Design review of the part built by this model. Coordinates are the model's own, in mm. Face numbers are marked on the shaded views. A direction names the side the tool comes from. Round coordinates to 2 decimals unless told otherwise and drop trailing zeros. Order: outer loops, then holes, each group sorted by start corner. A loop starts at its lowest first (then second) coordinate and runs counter-clockwise, first axis right, second up.
Autodesk Inventor part; units mm, degrees
ref_plane "YZ Plane" through (0, 0, 0) normal (1, 0, 0) x (0, 1, 0)
ref_plane "XZ Plane" through (0, 0, 0) normal (0, 1, 0) x (-1, 0, 0)
ref_plane "XY Plane" through (0, 0, 0) normal (0, 0, 1) x (1, 0, 0)
sketch "Sketch1" plane through (0, 0, 0) normal (0, 1, 0) x (-1, 0, 0)
  circle A0 centre (-11.43, -21.12) radius 0.25
  circle A1 centre (-11.43, -28.88) radius 0.25
  circle A2 centre (-9, -34.5) radius 1.25
  line L0 (11.43, -28.88) -> (-11.43, -28.88) construction
  circle A3 centre (11.43, -21.12) radius 0.25
  circle A4 centre (11.43, -28.88) radius 0.25
  arc A5 (-17.5, -24) -> (17.5, -24) centre (0, -24) ccw
  circle A6 centre (11.43, 2.12) radius 0.25
  circle A7 centre (-11.43, 9.88) radius 0.25
  circle A8 centre (11.43, 9.88) radius 0.25
  circle A9 centre (-9, 15.5) radius 1.25
  arc A10 (17.5, 5) -> (-17.5, 5) centre (0, 5) ccw
  circle A11 centre (-11.43, 2.12) radius 0.25
  circle A12 centre (12, -9.5) radius 1.25
  line L1 (17.5, -24) -> (17.5, 5)
  line L2 (11.43, -21.12) -> (11.43, 2.12) construction
  line L3 (0, -24) -> (0, 5) construction
  line L4 (-17.5, 5) -> (-17.5, -24)
  line L5 (-9, -34.5) -> (-9, 15.5) construction
  circle A13 centre (0, 0) radius 2.75
  point P0 (0, -41.5)
  point P1 (0, -28.88)
  point P2 (0, 22.5)
  point P3 (-9, -9.5)
  point P4 (11.43, -9.5)
  point P5 (0, -9.5)
  dimension "d0" = 17.5
  dimension "d2" = 5.5
  dimension "d3" = 64
  dimension "d4" = 2.5
  dimension "d5" = 12
  dimension "d6" = 50
  dimension "d7" = 9
  dimension "d8" = 22.86
  dimension "d9" = 7.76
  dimension "d10" = 7.76
  dimension "d11" = 23.24
  dimension "d12" = 0.5
  dimension "d13" = 9.5
extrude "Extrusion1" add sketch "Sketch1" against normal blind 9.2 contours A0 | A1 | A2 | A3 | A4 | L4 A10 L1 A5 | A6 | A7 | A8 | A9 | A11 | A12 | A13
chamfer "Chamfer1" distance 4 distance2 5 4 edges at (0, -9.2, 22.5) (-17.5, -9.2, -9.5) (0, -9.2, -41.5) (17.5, -9.2, -9.5) measured on face at (-5.8333, -9.2, -14.3333)
extrude "Extrusion2" add sketch "Sketch1" along normal blind 2.8 contours A0 | A1 | A3 | A4 | A6 | A7 | A8 | A11
extrude "Extrusion3" add sketch "Sketch1" along normal blind 3.8 contours A2 | A9 | A12
chamfer "Chamfer2" distance 0.2 angle 45 3 edges at (-10.75, 3.8, -9.5) (10.25, 3.8, 15.5) (10.25, 3.8, -34.5)
extrude "Extrusion4" add sketch "Sketch1" along normal blind 6.4 contours A13
chamfer "Chamfer3" distance 0.25 distance2 6.4 1 edges at (2.75, 6.4, 0) measured on face at (-0.9684, 6.4, -0.426)
sketch "Sketch3" plane through (0, 6.4, 0) normal (0, 1, 0) x (1, 0, 0)
  circle A0 centre (0, 0) radius 2
  dimension "d31" = 4
extrude "Extrusion5" add sketch "Sketch3" along normal blind 4.8
sketch "Sketch4" plane through (0, 11.2, 0) normal (0, 1, 0) x (1, 0, 0)
  circle A0 centre (0, 0) radius 1
  dimension "d34" = 2
extrude "Extrusion6" add sketch "Sketch4" along normal blind 6.2
chamfer "Chamfer4" distance 0.25 angle 45 1 edges at (-1, 17.4, 0)
properties part number "BKA" material "ABS Plastic"
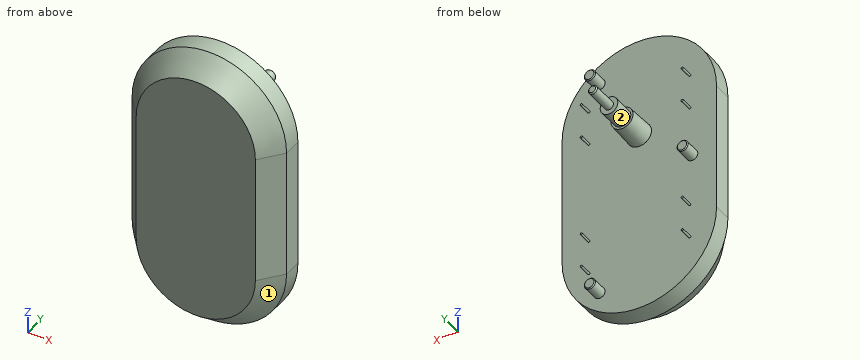
1) Take a section at B-B on y = -2. Give the boundary of the cut face in (x, z).
Results:
outline: (-17.5, -24) arc R17.5 ccw to (17.5, -24) - (17.5, 5) arc R17.5 ccw to (-17.5, 5) - close
2) For the marked faces 1 and 2, list the 3-axis set-ups (+Z, -Z, +X, -X, +Y, -Y) from which the entire face can be reached by the end or side of a thin tool; tool diameter is ignored.
Results:
face 1: -Z, -Y
face 2: +Y
3) To check wall thickness, follow line 1 along Y through (x, z) = (-2, -11); line 2 along X through (y, z) = (-7, -1.5); line 3 along Y through (x, z) = (14, -23.5) (3 decimals). State the ranges of each line that lie inside material, in increasing order.
Results:
line 1: y = -9.2 to 0
line 2: x = -15.26 to 15.26
line 3: y = -8.575 to 0
4) Take a section at A-A on z = -9.5. Give the boundary of the cut face in (x, y).
Results:
outline: (-17.5, -4.2) - (-13.5, -9.2) - (13.5, -9.2) - (17.5, -4.2) - (17.5, 0) - (-10.75, 0) - (-10.75, 3.6) - (-10.95, 3.8) - (-13.05, 3.8) - (-13.25, 3.6) - (-13.25, 0) - (-17.5, 0) - close
5) Clearance check with flat-ended pins moving along their axes: P1, Ø1, axis at x = 9.5, z = -34.5, coming from the +Y side; P2, Ø12, axis at x = -8, y = -4.5, coming from the -Z side; P3, Ø0.6, axis at x = -11.5, z = 10, coming from the +Y side; P4, Ø8, axis at y = 7, z = -16, coming from the +X side. State where each tip first meets the part, or that it passes through.
Results:
P1: stops at y = 3.8
P2: stops at z = -41.38
P3: stops at y = 2.8
P4: passes through
6) Take a section at C-C on y = 14.75. Give the boundary of the cut face in (x, z), plus the area to 3 significant figures.
Results:
outline: circle Ø2 at (0, 0)
area: 3.14 mm2
7) Take a section at D-D on y = -7. Give the boundary of the cut face in (x, z).
Results:
outline: (-15.26, -24) arc R15.26 ccw to (15.26, -24) - (15.26, 5) arc R15.26 ccw to (-15.26, 5) - close
